Build history of the part. All positions in model axes, mm. A direction names the side the tool comes from. Give positions to 0.01 mm unless a question says otherwise; leave off trailing zeros. Write each loop counter-clockwise with the first axis right and the second up, starting at its lowest first coordinate (ties: lowest second). Pieces come first, ordered by that corner, then holes. Notation, with made-up numbers: (-2, 58.25) -> (9, 58.25) arc R25 cw to (9, 77.25) -> close; hole circle Ø10 at (21, 70). An arc over 180 degrees is marked (long way). Put each result on its own line as item: value. Start each with the question number.
Item 1: Slice it at A-A, the plane y = -3.25. List the corners of the cut face in (x, z), plus the area to 3 significant figures.
Item 2: Two-plate mould, pull along Y, no slides. Class faces 1 (the flat face through (-9.303, 0, 0)), 2 (the flat face through (6.432, 3.628, 0.178)), 3 (the flat face through (0, -5.159, 0)), 4 (the flat face through (10.319, 0, 0)): pulls with the +Y half, pulls with the -Y half, needs draft (parallel to the pull), parting line crosses it, or undercut.
Item 3: Slice it at B-B, the plane x = 8.5. List the corners of the cut face in (y, z), plus the area to 3 significant figures.
Item 4: Slice it at D-D, the plane x = -0.25. List the corners of the cut face in (y, z), plus the area to 3 significant figures.
Item 5: Tool access for faces 5 (the flat face through (-5.556, 5, 0)), 6 (the flat face through (5.845, 3.642, 0.178)), 7 (the flat face through (8, 5.159, 0)): list every direction of +Z, -Z, +X, -X, +Y, -Y with a clear straight run to the whole face (end or side of a thin tool).
Item 6: Slice it at C-C, the plane z = -2.25. List the corners of the cut face in (x, y).
Item 7: Drill centre lines: line 1 along X through (y, z) = (-0.25, 1); line 2 along Y through (x, z) = (-7, -5.75); line 3 along X through (y, z) = (3.75, 9.5). Where is each one in solid material? Low to high.
```python
from build123d import *

# Parameters (mm, degrees)
BASE_EXTRUDE_DEPTH = 12.7


with BuildPart() as part:
    # Sketch1 → Base-Extrude (new, symmetric)
    with BuildSketch(Plane.XY):
        with BuildLine():
            Line((-5.55625, 5.159375), (-10.31875, 5.159375))
            Line((-10.31875, 5.159375), (-10.31875, -5.159375))
            Line((-10.31875, -5.159375), (10.31875, -5.159375))
            Line((10.31875, -5.159375), (10.31875, 5.159375))
            Line((10.31875, 5.159375), (5.55625, 5.159375))
            Line((5.55625, 5.159375), (5.55625, 4.143375))
            Line((5.55625, 4.143375), (6.142837874, 3.127375))
            Line((6.142837874, 3.127375), (6.729425747, 4.143375))
            Line((6.729425747, 4.143375), (8.79475, 4.143375))
            ThreePointArc((8.79475, 4.143375), (9.153960245, 3.994585245), (9.30275, 3.635375))
            Line((9.30275, 3.635375), (9.30275, -3.635375))
            ThreePointArc((9.30275, -3.635375), (9.153960245, -3.994585245), (8.79475, -4.143375))
            Line((8.79475, -4.143375), (-8.79475, -4.143375))
            ThreePointArc((-8.79475, -4.143375), (-9.153960245, -3.994585245), (-9.30275, -3.635375))
            Line((-9.30275, -3.635375), (-9.30275, 3.635375))
            ThreePointArc((-9.30275, 3.635375), (-9.153960245, 3.994585245), (-8.79475, 4.143375))
            Line((-8.79475, 4.143375), (-6.729425747, 4.143375))
            Line((-6.729425747, 4.143375), (-6.142837874, 3.127375))
            Line((-6.142837874, 3.127375), (-5.55625, 4.143375))
            Line((-5.55625, 4.143375), (-5.55625, 5.159375))
        make_face()
    extrude(amount=BASE_EXTRUDE_DEPTH, both=True)


solid = part.part
```
Values follow:
1. outline: (-10.32, -12.7) -> (-9.3, -12.7) -> (-9.3, 12.7) -> (-10.32, 12.7) -> close; (9.3, -12.7) -> (10.32, -12.7) -> (10.32, 12.7) -> (9.3, 12.7) -> close
1. area: 51.6 mm2
2. face 1: undercut
2. face 2: undercut
2. face 3: pulls with the -Y half
2. face 4: needs draft
3. outline: (-5.16, -12.7) -> (-4.14, -12.7) -> (-4.14, 12.7) -> (-5.16, 12.7) -> close; (4.14, -12.7) -> (5.16, -12.7) -> (5.16, 12.7) -> (4.14, 12.7) -> close
3. area: 51.6 mm2
4. outline: (-5.16, -12.7) -> (-4.14, -12.7) -> (-4.14, 12.7) -> (-5.16, 12.7) -> close
4. area: 25.8 mm2
5. face 5: +Z, -Z, +Y
5. face 6: +Z, -Z
5. face 7: +Z, -Z, +X, -X, +Y
6. outline: (-10.32, -5.16) -> (10.32, -5.16) -> (10.32, 5.16) -> (5.56, 5.16) -> (5.56, 4.14) -> (6.14, 3.13) -> (6.73, 4.14) -> (8.79, 4.14) arc R0.51 cw to (9.3, 3.64) -> (9.3, -3.64) arc R0.51 cw to (8.79, -4.14) -> (-8.79, -4.14) arc R0.51 cw to (-9.3, -3.64) -> (-9.3, 3.64) arc R0.51 cw to (-8.79, 4.14) -> (-6.73, 4.14) -> (-6.14, 3.13) -> (-5.56, 4.14) -> (-5.56, 5.16) -> (-10.32, 5.16) -> close
7. line 1: -10.32 to -9.3, 9.3 to 10.32
7. line 2: -5.16 to -4.14, 4.14 to 5.16
7. line 3: -10.32 to -9.29, -6.5 to -5.78, 5.78 to 6.5, 9.29 to 10.32
